Geometry check sheet. Reference: the model listing, model coordinates, mm. A direction names the side the tool comes from. Coordinates: 2 decimals unless noted, no trailing zeros. Order: outer loops, then holes, each group sorted by start corner. A loop starts at its lowest first (then second) coordinate and runs counter-clockwise, first axis right, second up.
```python
from build123d import *

# Parameters (mm, degrees)
BOSS_EXTRUDE1_DEPTH = 225
SKETCH3_W           = 30
SKETCH3_H           = 125
CUT_EXTRUDE1_DEPTH  = 225
SKETCH4_R           = 4.687343619
CUT_EXTRUDE2_DEPTH  = 225
CHAMFER1_SIZE       = 2


with BuildPart() as part:
    # Sketch1 → Boss-Extrude1 (new body)
    with BuildSketch(Plane.XY):
        Polygon((-39.755639098, 20.306390977), (5.244360902, 20.306390977), (5.244360902, -18.693609023), (3.744360902, -18.693609023), (3.744360902, 18.806390977), (-39.755639098, 18.806390977), align=None)
    extrude(amount=BOSS_EXTRUDE1_DEPTH)

    # Sketch3 → Cut-Extrude1 (cut)
    with BuildSketch(Plane(origin=(0, 20.306390977, 0), x_dir=(1, 0, 0), z_dir=(0, 1, 0))):
        with Locations((-24.755639098, -107.5)):
            Rectangle(SKETCH3_W, SKETCH3_H)
    extrude(amount=-CUT_EXTRUDE1_DEPTH, mode=Mode.SUBTRACT)

    # Sketch4 → Cut-Extrude2 (cut)
    with BuildSketch(Plane.ZY.offset(-3.744360902)):
        with Locations((5, 11.306390977)):
            Circle(SKETCH4_R)
        with Locations((220, 11.306390977)):
            Circle(SKETCH4_R)
    extrude(amount=-CUT_EXTRUDE2_DEPTH, mode=Mode.SUBTRACT)

    # Chamfer1
    chamfer1_edges = [part.edges().sort_by_distance(p)[0] for p in [
        (4.494360902, -18.693609023, 225),
        (-39.755639098, 19.556390977, 170),
        (-39.755639098, 19.556390977, 45),
        (-39.755639098, 19.556390977, 225),
        (4.494360902, -18.693609023, 0),
        (-39.755639098, 19.556390977, 0),
    ]]
    chamfer(chamfer1_edges, length=CHAMFER1_SIZE)


solid = part.part
```
Item 1: Thickness scan on line 1 along Y through (x, z) = (4, 5); line 2 along X through (y, z) = (-2.5, 197); line 3 along Y through (x, z) = (-3, 30.5). Record the ranges inside material, lowest first.
Item 2: Sectioned sample at B-B (x = -33). Record the cut outline in (y, z).
Item 3: Release check for a two-part mould opening along Z. For faces 3 (the face through (-7, 20, 0)), 4 (the face through (-7, 20, 225)), 5 (the face through (3.744, 0, 111)), 6 (the face through (4.484, 12.714, 9.471)) record: pulls with the +Z half, pulls with the -Z half, needs draft (parallel to the pull), parting line crosses it, or undercut.
Item 4: Sectioned sample at C-C (z = 148.5). Record the cut outline in (x, y), and give its area (4 significant figures).
Item 5: Sectioned sample at A-A (z = 220). Record the cut outline in (x, y), and give its area (3 significant figures).
Item 6: Tool access check on faces 1 (the face through (5.244, 1, 111)), 2 (the face through (-8, 18.806, 111)). Record the directions out of +Z, -Z, +X, -X, +Y, -Y that give a thin tool (end or side, any length) a straight path to the whole face; none if there is none.
Item 7: Sectioned sample at D-D (y = -2). Record the cut outline in (x, z), and give its area (4 significant figures).
Item 8: Depth check by flat-ended pin: P1, Ø12, axis at y = 11.31, z = 220, coming from the -X side; P2, Ø8, axis at x = -2.5, z = 196.5, coming from the -Y side; P3, Ø10, axis at x = -23.5, z = 53.5, coming from the -Y side. Enter the tip coordinate at first touch or a pass-through.
Geometry check:
1. line 1: y = -18.69 to 6.62, 15.99 to 20.31
1. line 2: x = 3.74 to 5.24
1. line 3: y = 18.81 to 20.31
2. outline: (18.81, 0) - (20.31, 0) - (20.31, 45) - (18.81, 45) - close; (18.81, 170) - (20.31, 170) - (20.31, 225) - (18.81, 225) - close
3. face 3: pulls with the -Z half
3. face 4: pulls with the +Z half
3. face 5: needs draft
3. face 6: undercut
4. outline: (-9.76, 18.81) - (3.74, 18.81) - (3.74, -18.69) - (5.24, -18.69) - (5.24, 20.31) - (-9.76, 20.31) - close
4. area: 78.75 mm2
5. outline: (-39.76, 18.81) - (3.74, 18.81) - (3.74, 15.99) - (5.24, 15.99) - (5.24, 20.31) - (-39.76, 20.31) - close; (3.74, -18.69) - (5.24, -18.69) - (5.24, 6.62) - (3.74, 6.62) - close
5. area: 110 mm2
6. face 1: +Z, -Z, +X, +Y, -Y
6. face 2: +Z, -Z, -X, -Y
7. outline: (3.74, 0) - (5.24, 0) - (5.24, 225) - (3.74, 225) - close
7. area: 337.5 mm2
8. P1: stops at x = 3.74
8. P2: stops at y = 18.81
8. P3: passes through
